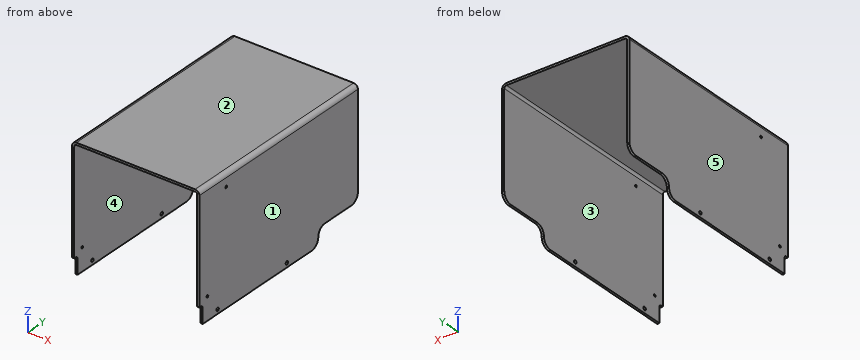
```python
from build123d import *

# Parameters (mm, degrees)
BOSS_EXTRUDE1_DEPTH = 609.6
FILLET1_R           = 6.35
FILLET2_R           = 12.7
SKETCH2_W           = 50.8
SKETCH2_H           = 12.7
CUT_EXTRUDE1_DEPTH  = 805.748204409
SKETCH4_W           = 50.8
SKETCH4_H           = 152.4
CUT_EXTRUDE2_DEPTH  = 805.748204409
SKETCH5_R           = 3.3782
CUT_EXTRUDE3_DEPTH  = 805.748204409
SKETCH6_R           = 4.7625
CUT_EXTRUDE4_DEPTH  = 805.748204409
FILLET3_R           = 25.4
FILLET4_R           = 6.35


with BuildPart() as part:
    # Sketch1 → Boss-Extrude1 (new body)
    with BuildSketch(Plane(origin=(0, 0, 0), x_dir=(1, 0, 0), z_dir=(0, 1, 0))):
        Polygon((0, 0), (0, -368.3), (374.65, -368.3), (374.65, 0), (368.3, 0), (368.3, -361.95), (6.35, -361.95), (6.35, 0), align=None)
    extrude(amount=BOSS_EXTRUDE1_DEPTH)

    # Fillet1
    fillet1_edges = [part.edges().sort_by_distance(p)[0] for p in [
        (6.35, 304.8, 361.95),
        (368.3, 304.8, 361.95),
    ]]
    fillet(fillet1_edges, radius=FILLET1_R)

    # Fillet2
    fillet2_edges = [part.edges().sort_by_distance(p)[0] for p in [
        (374.65, 304.8, 368.3),
        (0, 304.8, 368.3),
    ]]
    fillet(fillet2_edges, radius=FILLET2_R)

    # Sketch2 → Cut-Extrude1 (cut, through all)
    with BuildSketch(Plane(origin=(374.65, 0, 0), x_dir=(0, 0, -1), z_dir=(1, 0, 0))):
        with Locations((-25.4, 6.35)):
            Rectangle(SKETCH2_W, SKETCH2_H)
    extrude(amount=-CUT_EXTRUDE1_DEPTH, mode=Mode.SUBTRACT)

    # Sketch4 → Cut-Extrude2 (cut, through all)
    with BuildSketch(Plane(origin=(374.65, 0, 0), x_dir=(0, 0, -1), z_dir=(1, 0, 0))):
        with Locations((-25.4, 533.4)):
            Rectangle(SKETCH4_W, SKETCH4_H)
    extrude(amount=-CUT_EXTRUDE2_DEPTH, mode=Mode.SUBTRACT)

    # Sketch5 → Cut-Extrude3 (cut, through all)
    with BuildSketch(Plane(origin=(374.65, 0, 0), x_dir=(0, 0, -1), z_dir=(1, 0, 0))):
        with Locations((-330.2, 103.432077108)):
            Circle(SKETCH5_R)
        with Locations((-66.675, 30.736970621)):
            Circle(SKETCH5_R)
    extrude(amount=-CUT_EXTRUDE3_DEPTH, mode=Mode.SUBTRACT)

    # Sketch6 → Cut-Extrude4 (cut, through all)
    with BuildSketch(Plane(origin=(374.65, 0, 0), x_dir=(0, 0, -1), z_dir=(1, 0, 0))):
        with Locations((-12.7, 69.85)):
            Circle(SKETCH6_R)
        with Locations((-12.7, 336.55)):
            Circle(SKETCH6_R)
    extrude(amount=-CUT_EXTRUDE4_DEPTH, mode=Mode.SUBTRACT)

    # Fillet3
    fillet3_edges = [part.edges().sort_by_distance(p)[0] for p in [
        (3.175, 457.2, 0),
        (371.475, 457.2, 0),
        (371.475, 457.2, 50.8),
        (3.175, 457.2, 50.8),
        (3.175, 609.6, 50.8),
        (371.475, 609.6, 50.8),
    ]]
    fillet(fillet3_edges, radius=FILLET3_R - 0.0001)  # a hair under: the kernel refuses the full size

    # Fillet4
    fillet4_edges = [part.edges().sort_by_distance(p)[0] for p in [
        (371.475, 12.7, 50.8),
        (3.175, 12.7, 50.8),
    ]]
    fillet(fillet4_edges, radius=FILLET4_R)


solid = part.part
```
Read the model definition and answer for the solid it produces. Units are mm, in the model's axes. Face numbers are marked on the shaded views. A direction names the side the tool comes from. Give positions to 0.01 mm unless a question says otherwise; leave off trailing zeros. Write each loop counter-clockwise with the first axis right and the second up, starting at its lowest first coordinate (ties: lowest second). Pieces come first, ordered by that corner, then holes. Notation, with made-up numbers: M 0,47.25 L 55,47.25 A8 ccw 55,57.25 Z; hole C 20,82.25 d9. An arc over 180 degrees is marked long. Put each result on its own line as item: value. Start each with the question number.
1. The part is cut by section A-A, the plane z = 192.5. Give the vertices of the cut face in (x, y).
2. The part is cut by section D-D, the plane z = 38. Give the vertices of the cut face in (x, y), and give its area (3 significant figures).
3. The part is cut by section B-B, the plane y = 167. Give the vertices of the cut face in (x, z), and give its area (3 significant figures).
4. The part is cut by section C-C, the plane x = 28.5. Give the vertices of the cut face in (y, z).
5. For a pull along X with two mould halves and no side action, classify the marked faces 1, 2 and 3 as released by +X, released by -X, zero draft, split by the parting line, or undercut.
6. Which of the six approach directions +Z, -Z, +X, -X, +Y, -Y give full straight-line access (tool end or side, diameter ignored) to the marked faces 4 and 5?
7. Consider line 1 along X through (y, z) = (339, 304); line 2 along Z through (x, y) = (17, 222.5); line 3 along Z through (x, y) = (5, 69). Determine where each line is inside the solid, lowest interval first.
8. Each of these flat-tipped pins is pushed along its axis until it touches: pin 1 Ø1.9 at (x, y) = (2.5, 530.5) entering from -Z; pin 2 Ø2 at (x, y) = (184, 425) entering from -Z; pin 3 Ø15 at (y, z) = (69.85, 12.7) entering from -X; pin 4 Ø7 at (x, z) = (371.5, 22) entering from -Y. Where does it stop, or does it pass through?
Final values:
1. outline: M 0,0 L 6.35,0 L 6.35,609.6 L 0,609.6 Z; M 368.3,0 L 374.65,0 L 374.65,609.6 L 368.3,609.6 Z
2. outline: M 0,12.7 L 6.35,12.7 L 6.35,460.55 L 0,460.55 Z; M 368.3,12.7 L 374.65,12.7 L 374.65,460.55 L 368.3,460.55 Z
2. area: 5,690 mm²
3. outline: M 0,0 L 6.35,0 L 6.35,355.6 A6.35 cw 12.7,361.95 L 361.95,361.95 A6.35 cw 368.3,355.6 L 368.3,0 L 374.65,0 L 374.65,355.6 A12.7 ccw 361.95,368.3 L 12.7,368.3 A12.7 ccw 0,355.6 Z
3. area: 6,920 mm²
4. outline: M 0,361.95 L 609.6,361.95 L 609.6,368.3 L 0,368.3 Z
5. face 1: released by +X
5. face 2: zero draft
5. face 3: undercut
6. face 4: -Z, +Y, -Y
6. face 5: +Z, -Z, -X, +Y, -Y
7. line 1: x = 0 to 6.35, 368.3 to 374.65
7. line 2: z = 361.95 to 368.3
7. line 3: z = 0 to 8.01, 17.39 to 365.7
8. pin 1: stops at z = 50.8
8. pin 2: stops at z = 361.95
8. pin 3: stops at x = 0
8. pin 4: stops at y = 12.7
